Verification items for the finished model (mm, model axes). Coordinates: 2 decimals unless noted, no trailing zeros. Write each loop counter-clockwise with the first axis right and the second up, starting at its lowest first coordinate (ties: lowest second). Pieces come first, ordered by that corner, then holes. Notation, with made-up numbers: (82, -38) -> (107, -38) arc R30 cw to (107, 1) -> close; hole circle Ø10 at (72, 70). An arc over 180 degrees is marked (long way). Write item = value, one per line. Start each with the question number.
(1) Section check A-A (y = -5). Record the cut outline in (x, z) (3 decimals), plus the area to 3 significant figures.
(2) Gauge pin test, flat ends, axial feed: pin 1 Ø8 at (x, y) = (-48.5, -2.5) entering from +Z; pin 2 Ø1.5 at (x, y) = (-79.5, -2.5) entering from +Z; pin 3 Ø4 at (x, z) = (-4.6, -18) entering from -Y; pin 4 Ø5 at (x, z) = (-140.8, -30.4) entering from -Y. Record the tip position at first contact, or that the pin passes through.
(3) Section check D-D (x = -132). Record the cut outline in (y, z).
(4) Section check B-B (x = -170). Record the cut outline in (y, z).
(5) Section check C-C (z = -53.6). Record the cut outline in (x, y), plus the area to 3 significant figures.
(6) Material ranges on probe 1 along X at (y, z) = (1.2, -105); probe 2 along X at (y, z) = (-18, -56.5); probe 3 along Y at (x, z) = (-105.5, -54.5), recorded low to high. Write a range as [from, to].
Autodesk Inventor part; units mm, degrees
ref_plane "YZ Plane" through (0, 0, 0) normal (1, 0, 0) x (0, 1, 0)
ref_plane "XZ Plane" through (0, 0, 0) normal (0, 1, 0) x (-1, 0, 0)
ref_plane "XY Plane" through (0, 0, 0) normal (0, 0, 1) x (1, 0, 0)
sketch "Szkic1" plane through (0, 0, 0) normal (0, 1, 0) x (-1, 0, 0)
  point P0 (0, 0)
sketch "Szkic2" plane through (0, 0, 0) normal (0, 1, 0) x (-1, 0, 0)
  line L0 (0, 0) -> (140, 0)
  line L1 (190, -18) -> (190, -66)
  line L2 (140, -84) -> (0, -84)
  line L3 (0, -84) -> (0, 0)
  line L4 (140, 0) -> (190, -18)
  line L5 (190, -66) -> (140, -84)
  circle A0 centre (170, -30.4) radius 2.1
  circle A1 centre (170, -53.6) radius 2.1
  line L6 (190, -42) -> (110.3864, -42)
  circle A2 centre (140.8, -30.4) radius 2.1
  circle A3 centre (140.8, -53.6) radius 2.1
  circle A4 centre (10.75, 21) radius 1.25
  circle A5 centre (10.75, -105) radius 1.25
  circle A6 centre (28, 21) radius 1.25
  circle A7 centre (28, -105) radius 1.25
  line L7 (0, -84) -> (40, -84)
  line L8 (40, -84) -> (40, -109)
  line L9 (40, -109) -> (0, -109)
  line L10 (0, -109) -> (0, -84)
  line L11 (0, 0) -> (40, 0)
  line L12 (40, 0) -> (40, 25)
  line L13 (40, 25) -> (0, 25)
  line L14 (0, 25) -> (0, 0)
  circle A8 centre (4.5993, -66) radius 2.1
  circle A9 centre (4.5993, -18) radius 2.1
  point P0 (20, -84)
  point P1 (20, -109)
  point P2 (40, -96.5)
  point P3 (40, 12.5)
  point P4 (0, 12.5)
  point P5 (40, 0)
  point P6 (40, -84)
  dimension "d3" = 48
  dimension "d4" = 140
  dimension "d5" = 84
  dimension "d6" = 4.2
  dimension "d7" = 4.2
  dimension "d8" = 23.2
  dimension "d9" = 11.6
  dimension "d10" = 4.2
  dimension "d11" = 29.2
  dimension "d12" = 4.2
  dimension "d13" = 2.5
  dimension "d14" = 2.5
  dimension "d15" = 2.5
  dimension "d16" = 2.5
  dimension "d17" = 28
  dimension "d18" = 28
  dimension "d19" = 42
  dimension "d20" = 50
  dimension "d21" = 50
  dimension "d46" = 17.25
  dimension "d47" = 17.25
  dimension "d73" = 23.2
  dimension "d74" = 29.2
  dimension "d78" = 20
  dimension "d79" = 20
  dimension "d80" = 49.2
  dimension "d83" = 25
  dimension "d84" = 40
  dimension "d85" = 25
  dimension "d86" = 40
  dimension "d87" = 4
  dimension "d88" = 4
  dimension "d89" = 4
  dimension "d90" = 4
  dimension "d91" = 4.2
  dimension "d92" = 4.2
  dimension "d93" = 18
  dimension "d94" = 18
extrude "Wyciągnięcie proste1" add sketch "Szkic2" along normal blind 2
sketch "Szkic3" plane through (-190, 0, -66) normal (-1, 0, 0) x (0, 0, 1)
  line L0 (0, 2) -> (48, 2)
  line L1 (48, 2) -> (0, 2)
  line L2 (0, 2) -> (0, -19)
  line L3 (0, -19) -> (48, -19)
  line L4 (48, -19) -> (48, 2)
  circle A0 centre (37.195, -10) radius 8
  line L5 (0, 0) -> (48, 0)
  circle A1 centre (10.805, -10) radius 8
  circle A2 centre (46.6, -1.4) radius 1
  circle A3 centre (46.6, -17.6) radius 1
  circle A4 centre (1.4, -17.6) radius 1
  circle A5 centre (1.4, -1.4) radius 1
  point P0 (66, 0)
  dimension "d24" = 48
  dimension "d25" = 21
  dimension "d26" = 10
  dimension "d28" = 16
  dimension "d29" = 10
  dimension "d31" = 16
  dimension "d32" = 1.4
  dimension "d33" = 1.4
  dimension "d34" = 1.4
  dimension "d35" = 1.4
  dimension "d36" = 1.4
  dimension "d37" = 1.4
  dimension "d38" = 1.4
  dimension "d39" = 1.4
  dimension "d40" = 2
  dimension "d41" = 2
  dimension "d42" = 2
  dimension "d43" = 2
  dimension "d75" = 26.39
  dimension "d76" = 10.805
  dimension "d77" = 10.805
extrude "Wyciągnięcie proste2" add sketch "Szkic3" against normal blind 2 contours L5 L4 L3 L2
sketch "Szkic4" plane through (0, 0, 0) normal (0, -1, 0) x (1, 0, 0)
  line L0 (-140, 0) -> (0, 0)
  line L1 (-40, -84) -> (-140, -84)
  line L2 (-55, -84) -> (-55, 0)
  line L3 (0, 0) -> (0, -109)
  line L4 (-125, -84) -> (-125, 0)
  circle A0 centre (-65.9, -29.27) radius 1.375
  circle A1 centre (-114.07, -28) radius 1.375
  circle A2 centre (-81.25, -79.81) radius 1.375
  point P0 (0, -84)
  point P1 (-70, 0)
  dimension "d60" = 55
  dimension "d61" = 70
  dimension "d62" = 2.75
  dimension "d63" = 10.9
  dimension "d64" = 29.27
  dimension "d65" = 2.75
  dimension "d66" = 28
  dimension "d67" = 59.07
  dimension "d68" = 79.81
  dimension "d69" = 2.75
  dimension "d70" = 26.25
extrude "Wyciągnięcie proste3" add sketch "Szkic4" along normal blind 16 contours A0 | A1 | A2
properties part number "robocik"
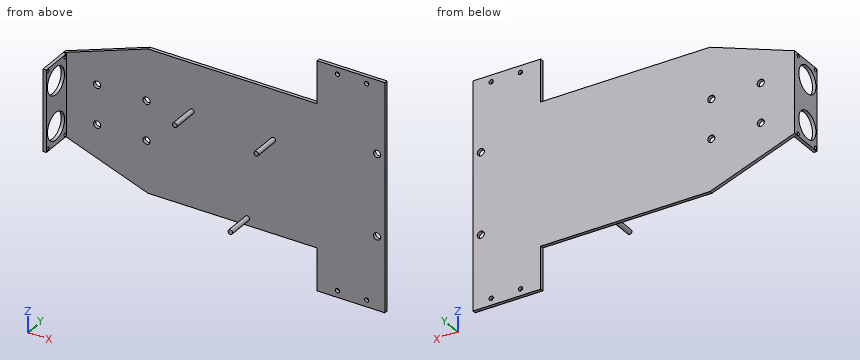
Response:
q1.outline = (-190, -66) -> (-188, -66) -> (-188, -61.44) -> (-190, -61.44) -> close; (-190, -48.95) -> (-188, -48.95) -> (-188, -35.05) -> (-190, -35.05) -> close; (-190, -22.56) -> (-188, -22.56) -> (-188, -18) -> (-190, -18) -> close; circle Ø2.75 at (-114.07, -28); circle Ø2.75 at (-81.25, -79.81); circle Ø2.75 at (-65.9, -29.27)
q1.area = 63.9 mm2
q2.pin_1 = 0
q2.pin_2 = -78.87
q2.pin_3 = through
q2.pin_4 = 0
q3.outline = (0, -84) -> (2, -84) -> (2, 0) -> (0, 0) -> close
q4.outline = (0, -73.2) -> (2, -73.2) -> (2, -55.7) -> (0, -55.7) -> close; (0, -51.5) -> (2, -51.5) -> (2, -32.5) -> (0, -32.5) -> close; (0, -28.3) -> (2, -28.3) -> (2, -10.8) -> (0, -10.8) -> close
q5.outline = (-190, -19) -> (-188, -19) -> (-188, -17.84) -> (-190, -17.84) -> close; (-190, -2.16) -> (-188, -2.16) -> (-188, 0) -> (-172.1, 0) -> (-172.1, 2) -> (-190, 2) -> close; (-167.9, 0) -> (-142.9, 0) -> (-142.9, 2) -> (-167.9, 2) -> close; (-138.7, 0) -> (0, 0) -> (0, 2) -> (-138.7, 2) -> close
q5.area = 370 mm2
q6.probe_1 = [-40, -29.25], [-26.75, -12], [-9.5, 0]
q6.probe_2 = [-190, -188]
q6.probe_3 = [0, 2]
